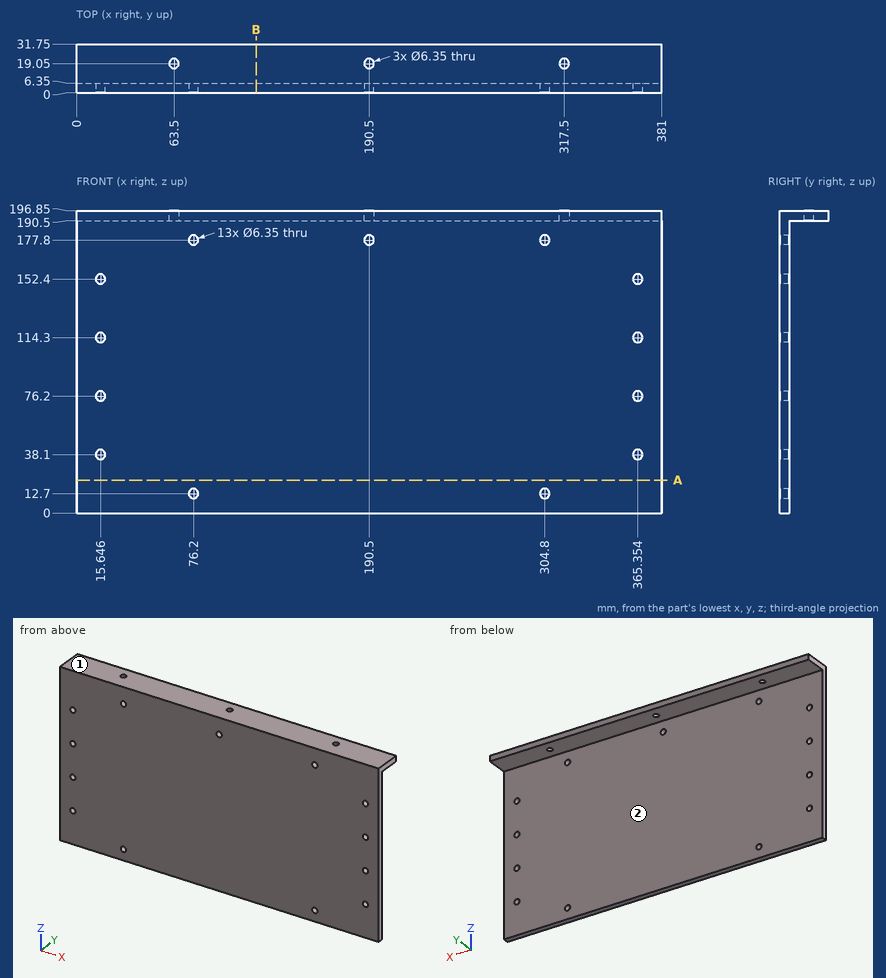
Geometry check sheet. Reference: drawing and pictorial views, mm from the part's lowest x, y, z. A direction names the side the tool comes from. Coordinates: 2 decimals unless noted, no trailing zeros. Loops run counter-clockwise (first coordinate to the right, second up) from the corner with the lowest first, then second, coordinate; pieces in that order, holes last. Notation, with made-up numbers: (8, 72.5) -> (67, 72.5) arc R24 ccw to (67, 105.5) -> close; hole circle Ø5 at (29.5, 83). An arc over 180 degrees is marked (long way). Write item = value, one per line. Start each with the question number.
1. Section check B-B on x = 117. Record the cut outline in (y, z).
2. Depth check by flat-ended pin: P1, Ø10, axis at x = 365.35, z = 76.2, coming from the +Y side; P2, Ø2, axis at x = 92, y = 13, coming from the -Z side. Enter the tip coordinate at first touch or a pass-through.
3. Tool access check on the marked faces 1 and 2. Record the directions out of +Z, -Z, +X, -X, +Y, -Y that give a thin tool (end or side, any length) a straight path to the whole face; none if there is none.
4. Section check A-A on z = 21.5. Record the cut outline in (x, y).
5. Material ranges on line 1 (X direction, y = 3, z = 114) (1 decimal); line 2 (X direction, y = 3, z = 12); line 3 (Z direction, x = 76, y = 4), recorded low to high.
Responses:
q1.outline = (0, 0) -> (6.35, 0) -> (6.35, 190.5) -> (31.75, 190.5) -> (31.75, 196.85) -> (0, 196.85) -> close
q2.P1 = 6.35
q2.P2 = 190.5
q3.face_1 = +Z, +X, -X, +Y, -Y
q3.face_2 = -Z, +X, -X, +Y
q4.outline = (0, 0) -> (381, 0) -> (381, 6.35) -> (0, 6.35) -> close
q5.line_1 = 0 to 12.5, 18.8 to 362.2, 368.5 to 381
q5.line_2 = 0 to 73.1, 79.3 to 301.7, 307.9 to 381
q5.line_3 = 0 to 9.53, 15.87 to 174.63, 180.97 to 196.85
